Design review of the part built by this model. Coordinates are the model's own, in mm. A direction names the side the tool comes from. Coordinates: 2 decimals unless noted, no trailing zeros. Write each loop counter-clockwise with the first axis right and the second up, starting at its lowest first coordinate (ties: lowest second). Pieces come first, ordered by that corner, then holes. Notation, with made-up numbers: M 82.5,43.5 L 93.5,43.5 A29 cw 93.5,66.5 Z; hole C -6.5,-35 d9. An arc over 180 degrees is marked long. One line per question, with ' | ' between items.
Autodesk Inventor part; units mm, degrees
ref_plane "YZ Plane" through (0, 0, 0) normal (1, 0, 0) x (0, 1, 0)
ref_plane "XZ Plane" through (0, 0, 0) normal (0, 1, 0) x (-1, 0, 0)
ref_plane "XY Plane" through (0, 0, 0) normal (0, 0, 1) x (1, 0, 0)
sketch "Sketch1" plane through (0, 0, 0) normal (0, 1, 0) x (-1, 0, 0)
  line L0 (0, 0) -> (787.4, 0)
  line L1 (787.4, 0) -> (787.4, -533.4)
  line L2 (787.4, -533.4) -> (0, -533.4)
  line L3 (0, -533.4) -> (0, 0)
  dimension "d0" = 787.4
  dimension "d1" = 533.4
extrude "Extrusion1" add sketch "Sketch1" along normal blind 25.4
sketch "Sketch2" plane through (0, 25.4, 0) normal (0, 1, 0) x (1, 0, 0)
  line L0 (-787.4, 0) -> (0, 0)
  line L1 (-787.4, 533.4) -> (-787.4, 0)
  line L2 (0, 0) -> (-787.4, 0)
  line L3 (-787.4, 0) -> (-787.4, 12.7)
  line L4 (-787.4, 12.7) -> (0, 12.7)
  line L5 (0, 12.7) -> (0, 0)
  line L6 (0, 533.4) -> (-787.4, 533.4)
  line L7 (0, 0) -> (0, 533.4)
  line L8 (-787.4, 533.4) -> (0, 533.4)
  line L9 (0, 533.4) -> (0, 520.7)
  line L10 (0, 520.7) -> (-787.4, 520.7)
  line L11 (-787.4, 520.7) -> (-787.4, 533.4)
  line L12 (-787.4, 533.4) -> (-762, 533.4)
  line L13 (-762, 533.4) -> (-762, 0)
  line L14 (-762, 0) -> (-787.4, 0)
  line L15 (-787.4, 0) -> (-787.4, 533.4)
  dimension "d4" = 12.7
  dimension "d5" = 12.7
  dimension "d6" = 25.4
extrude "Extrusion2" add sketch "Sketch2" along normal blind 50.8 contours L1 L4 L13 L0 | L13 L4 L5 L0 | L1 L10 L13 L4 | L1 L6 L13 L10 | L13 L6 L7 L10
sketch "Sketch3" plane through (0, 25.4, 0) normal (0, 1, 0) x (1, 0, 0)
  line L0 (0, 533.4) -> (-787.4, 533.4) construction
  line L1 (0, 533.4) -> (0, 520.7) construction
  line L2 (0, 533.4) -> (0, 0) construction
  line L3 (0, 12.7) -> (0, 520.7) construction
  line L4 (0, 520.7) -> (0, 495.3) construction
  line L5 (-762, 520.7) -> (-762, 12.7) construction
  line L6 (-762, 520.7) -> (-762, 495.3) construction
  line L7 (0, 520.7) -> (-762, 520.7) construction
  line L8 (-762, 520.7) -> (-762, 419.1) construction
  line L9 (-762, 520.7) -> (-660.4, 520.7) construction
  arc A0 (-660.4, 520.7) -> (-762, 419.1) centre (-660.4, 419.1) ccw construction
  line L10 (0, 495.3) -> (-660.4, 495.3)
  line L11 (-660.4, 495.3) -> (-660.4, 482.6)
  line L12 (-660.4, 482.6) -> (0, 482.6)
  line L13 (0, 482.6) -> (0, 495.3)
  arc A1 (-660.4, 520.7) -> (-762, 419.1) centre (-660.4, 419.1) ccw
  line L14 (-762, 419.1) -> (-762, 520.7)
  line L15 (-762, 520.7) -> (-660.4, 520.7)
  dimension "d9" = 12.7
  dimension "d10" = 25.4
  dimension "d11" = 25.4
  dimension "d12" = 101.6
  dimension "d13" = 101.6
  dimension "d14" = 12.7
extrude "Extrusion3" add sketch "Sketch3" along normal blind 50.8
sketch "Sketch4" plane through (0, 25.4, 0) normal (0, 1, 0) x (1, 0, 0)
  line L0 (0, 12.7) -> (-762, 12.7) construction
  line L1 (-762, 12.7) -> (-654.2369, 120.4631) construction
  line L2 (-762, 12.7) -> (-609.6, 12.7) construction
  line L3 (-762, 419.1) -> (-762, 12.7)
  arc A0 (-762, 120.4631) -> (-654.2369, 12.7) centre (-654.2369, 120.4631) ccw
  line L4 (-654.2369, 12.7) -> (-762, 12.7)
  line L5 (-762, 120.4631) -> (-762, 12.7)
  point P0 (0, 0)
  dimension "d18" = 152.4
  dimension "d19" = 45
extrude "Extrusion4" add sketch "Sketch4" along normal blind 50.8
sketch "Sketch6" plane through (0, 76.2, 0) normal (0, 1, 0) x (1, 0, 0)
  line L0 (-660.4, 482.6) -> (0, 482.6)
  line L1 (-254.5688, 482.6) -> (-254.5688, 495.3)
  line L2 (0, 495.3) -> (-660.4, 495.3)
  line L3 (-254.5688, 482.6) -> (-305.3688, 482.6)
  line L4 (-305.3688, 482.6) -> (-305.3688, 495.3)
  line L5 (-305.3688, 495.3) -> (-254.5688, 495.3)
  point P0 (0, 0)
  dimension "d22" = 50.8
extrude "Extrusion5" cut sketch "Sketch6" against normal blind 50.8
sketch "Sketch8" plane through (0, 76.2, 0) normal (0, 1, 0) x (1, 0, 0)
  line L0 (-305.3688, 482.6) -> (-660.4, 482.6)
  line L1 (-660.4, 482.6) -> (-635, 482.6)
  line L2 (-635, 482.6) -> (-635, 495.3)
  line L3 (-305.3688, 495.3) -> (-660.4, 495.3)
  line L4 (-660.4, 495.3) -> (-635, 495.3)
  line L5 (-660.4, 482.6) -> (-660.4, 495.3)
  line L6 (-660.4, 482.6) -> (-660.4, 495.3)
  point P0 (0, 0)
  dimension "d26" = 25.4
extrude "Extrusion6" cut sketch "Sketch8" against normal blind 50.8
sketch "Sketch7" plane through (0, 25.4, 0) normal (0, 1, 0) x (1, 0, 0)
  line L0 (-254.5688, 495.3) -> (-279.9688, 520.7) construction
  line L1 (0, 520.7) -> (-660.4, 520.7) construction
  line L2 (-254.5688, 495.3) -> (-218.6478, 495.3) construction
  point P0 (0, 0)
  dimension "d25" = 135
sketch "Sketch9" plane through (0, 25.4, 0) normal (0, 1, 0) x (1, 0, 0)
  line L0 (0, 520.7) -> (-660.4, 520.7) construction
  line L1 (-635, 495.3) -> (-305.3688, 495.3) construction
  line L2 (-660.4, 520.7) -> (-635, 495.3) construction
  point P0 (0, 0)
sketch "Sketch10" plane through (0, 25.4, 0) normal (0, 1, 0) x (1, 0, 0)
  line L0 (-635, 482.6) -> (-305.3688, 482.6) construction
  line L1 (-635, 482.6) -> (-635, 444.5) construction
  line L2 (-635, 444.5) -> (-635, 419.1) construction
  line L3 (-635, 419.1) -> (-635, 381) construction
  line L4 (-635, 381) -> (-635, 355.6) construction
  line L5 (-635, 355.6) -> (-558.8, 355.6)
  line L6 (-558.8, 355.6) -> (-558.8, 381)
  line L7 (-558.8, 381) -> (-635, 381)
  line L8 (-635, 381) -> (-635, 355.6)
  line L9 (-635, 419.1) -> (-558.8, 419.1)
  line L10 (-558.8, 419.1) -> (-558.8, 444.5)
  line L11 (-558.8, 444.5) -> (-635, 444.5)
  line L12 (-635, 444.5) -> (-635, 419.1)
  point P0 (0, 0)
  dimension "d29" = 38.1
  dimension "d30" = 25.4
  dimension "d31" = 38.1
  dimension "d32" = 25.4
  dimension "d33" = 76.2
extrude "Extrusion7" add sketch "Sketch10" along normal blind 50.8
sketch "Sketch11" plane through (0, 25.4, 0) normal (0, 1, 0) x (1, 0, 0)
  line L0 (0, 12.7) -> (0, 247.65) construction
  line L1 (0, 247.65) -> (-101.6, 247.65) construction
  line L2 (-101.6, 247.65) -> (-101.6, 209.55) construction
  line L3 (-101.6, 209.55) -> (-101.6, 133.35) construction
  line L4 (-101.6, 133.35) -> (-155.4815, 79.4685) construction
  line L5 (-155.4815, 79.4685) -> (-231.6815, 79.4685) construction
  line L6 (-101.6, 247.65) -> (-101.6, 361.95) construction
  line L7 (-101.6, 361.95) -> (-155.4815, 415.8315) construction
  line L8 (-155.4815, 415.8315) -> (-231.6815, 415.8315) construction
  line L9 (-155.4815, 79.4685) -> (-101.6, 133.35)
  line L10 (-101.6, 133.35) -> (-76.2, 133.35)
  line L11 (-76.2, 133.35) -> (-155.4815, 54.0685)
  line L12 (-155.4815, 54.0685) -> (-231.6815, 54.0685)
  line L13 (-231.6815, 54.0685) -> (-231.6815, 79.4685)
  line L14 (-231.6815, 79.4685) -> (-155.4815, 79.4685)
  line L15 (-101.6, 361.95) -> (-76.2, 361.95)
  line L16 (-76.2, 361.95) -> (-155.4815, 441.2315)
  line L17 (-155.4815, 441.2315) -> (-231.6815, 441.2315)
  line L18 (-231.6815, 441.2315) -> (-231.6815, 415.8315)
  line L19 (-155.4815, 415.8315) -> (-231.6815, 415.8315)
  line L20 (-155.4815, 415.8315) -> (-101.6, 361.95)
  point P0 (0, 0)
  dimension "d36" = 234.95
  dimension "d37" = 101.6
  dimension "d38" = 38.1
  dimension "d39" = 76.2
  dimension "d40" = 76.2
  dimension "d41" = 135
  dimension "d42" = 76.2
  dimension "d43" = 114.3
  dimension "d44" = 76.2
  dimension "d45" = 135
  dimension "d46" = 25.4
extrude "Extrusion8" add sketch "Sketch11" along normal blind 50.8
sketch "Sketch12" plane through (0, 25.4, 0) normal (0, 1, 0) x (1, 0, 0)
  line L0 (0, 12.7) -> (0, 482.6) construction
  line L1 (0, 12.7) -> (0, 254) construction
  line L2 (0, 254) -> (-304.8, 254) construction
  circle A0 centre (-304.8, 254) radius 76.2
  point P0 (0, 0)
  dimension "d49" = 241.3
  dimension "d50" = 304.8
  dimension "d51" = 152.4
emboss "Emboss1" sketch "Sketch12" operation cut depth 12.7 direction (0, -1, 0)
properties part number "Playfield"
1. Take a section at D-D (x = -713). Write out the cut boundary in (y, z), then the cut area to 3 significant figures.
Answer sheet:
outline: M 0,-533.4 L 76.2,-533.4 L 76.2,-506.02 L 25.4,-506.02 L 25.4,-30.13 L 76.2,-30.13 L 76.2,0 L 0,0 Z | area: 16,500 mm^2
2. Tool access review of faces 4 (the face through (-597, 50, -419.1)), 5 (the face through (-166, 76.2, -79)), 6 (the face through (-193, 50, -54.068)): name each direction out of +Z, -Z, +X, -X, +Y, -Y from which nothing blocks a thin tool from reaching the whole face with its end or side.
Answer sheet:
face 4: +Y | face 5: +Z, -Z, +X, -X, +Y | face 6: +X, +Y
3. Take a section at A-A (x = -489.5). Write out the cut boundary in (y, z), then the cut area to 3 significant figures.
Answer sheet:
outline: M 0,-533.4 L 76.2,-533.4 L 76.2,-520.7 L 25.4,-520.7 L 25.4,-495.3 L 76.2,-495.3 L 76.2,-482.6 L 25.4,-482.6 L 25.4,-12.7 L 76.2,-12.7 L 76.2,0 L 0,0 Z | area: 15,500 mm^2
4. Draft analysis for pull direction X (two halves, no side actions). For faces 1 (the face through (-269.638, 19.139, -186.397)), 2 (the face through (-166, 76.2, -416)), 3 (the face through (0, 18, -288)), state which applies: pulls with the +X half, pulls with the -X half, needs draft (parallel to the pull), parting line crosses it, or undercut.
Answer sheet:
face 1: undercut | face 2: needs draft | face 3: pulls with the +X half
5. Insertion check: pin 1 Ø12 at (y, z) = (38.5, -323) entering from +X; pin 2 Ø2 at (y, z) = (41.5, -394) entering from +X; pin 3 Ø1 at (y, z) = (35, -443) entering from +X. Each pin has a flat end and moves straight along its axis. Give the tip position at first contact, or say it passes through.
Answer sheet:
pin 1: x = -762 | pin 2: x = -107.25 | pin 3: x = -558.8
6. To check wall thickness, follow line 1 along Z through (x, y) = (-460.5, 57.5); line 2 along Z through (x, y) = (-304, 19); line 3 along X through (y, z) = (19.75, -254). State the ranges of each line that lie inside material, in increasing order. Write a range as [from, to].
Answer sheet:
line 1: [-533.4, -520.7], [-495.3, -482.6], [-12.7, 0] | line 2: [-533.4, -330.2], [-177.8, 0] | line 3: [-787.4, -381], [-228.6, 0]
7. Take a section at B-B (y = 52). Count the separate pieces of the cut face and the enclosed holes in it, then the cut area to 3 significant figures.
Answer sheet:
separate pieces: 7 | enclosed holes: 0 | area: 56,200 mm^2
8. Take a section at C-C (z = -254). Write out the cut boundary in (x, y), then the cut area to 3 significant figures.
Answer sheet:
outline: M -787.4,0 L 0,0 L 0,25.4 L -228.6,25.4 L -228.6,12.7 L -381,12.7 L -381,25.4 L -762,25.4 L -762,76.2 L -787.4,76.2 Z | area: 19,400 mm^2
